```python
from build123d import *

# Parameters (mm, degrees)
F0_R     = 3
F1_DEPTH = 8
F3_DEPTH = 3
F4_R     = 2
F5_DEPTH = 25
F6_SIZE  = 0.99999
F7_R     = 4
F8_DEPTH = 1.5


# Not quite as in the source:
# - a fillet or chamfer is up to 0.001 mm smaller than in the source, because OpenCascade refuses the exact size


with BuildPart() as f1:
    # F0 (on Front) → F1 (new body)
    with BuildSketch(Plane.XZ):
        Circle(F0_R)
    extrude(amount=F1_DEPTH)

    # F2 (on face) → F3 (cut)
    with BuildSketch(Plane.XZ.offset(8)):
        Polygon((2, 1.1547005384), (0, 2.3094010768), (-2, 1.1547005384), (-2, -1.1547005384), (0, -2.3094010768), (2, -1.1547005384), align=None)
    extrude(amount=-F3_DEPTH, mode=Mode.SUBTRACT)

    # F4 (on face) → F5 (cut)
    with BuildSketch(Plane.XZ.offset(5)):
        Circle(F4_R)
    extrude(amount=-F5_DEPTH, mode=Mode.SUBTRACT)

    # F6 (size 1 in the source; OpenCascade refuses exactly that, so slightly less here)
    f6_edges = [f1.edges().sort_by_distance(p)[0] for p in [
        (-3, 0, 0),
    ]]
    chamfer(f6_edges, length=F6_SIZE)

    # F7 (on face) → F8 (join)
    with BuildSketch(Plane.XZ.offset(8)):
        Circle(F7_R)
        Polygon((2, 1.1547005384), (2, -1.1547005384), (0, -2.3094010768), (-2, -1.1547005384), (-2, 1.1547005384), (0, 2.3094010768), align=None, mode=Mode.SUBTRACT)
    extrude(amount=F8_DEPTH)


solid = f1.part
```
Could you check a few things on this model? Use its own coordinates, in mm. A direction names the side the tool comes from. Round coordinates to 2 decimals unless told otherwise and drop trailing zeros. Write each loop counter-clockwise with the first axis right and the second up, starting at its lowest first coordinate (ties: lowest second). Pieces come first, ordered by that corner, then holes.
(1) Suppose I cut it at A-A on y = -0.5. Write out the boundary of the cut face in (x, z).
Findings below:
outline: circle Ø5 at (0, 0); hole circle Ø4 at (0, 0)
(2) Thinking about a two-plate mould opening in X: for faces 1 (the face through (1, -9.5, 2)), 2 (the face through (2, -7, 0)), 3 (the face through (-0.867, -8.74, -3.905)), which applies, +X half, -X half, draft (parallel to the pull), parting line (faces both ways), or undercut?
Findings below:
face 1: draft
face 2: undercut
face 3: parting line
(3) Which directions (+Z, -Z, +X, -X, +Y, -Y) give clear straight access to the entire face, cutting with the end or side of a thin tool? Please do faces 4 (the face through (-3, -4, 0)), 5 (the face through (-2, -7, 0)), 6 (the face through (0, -3, -2)).
Findings below:
face 4: +Y
face 5: -Y
face 6: +Y, -Y
(4) If I drill on probe 1 along Z at (x, y) = (0, -3.3); probe 2 along Y at (x, z) = (2.75, -1.75); probe 3 along X at (y, z) = (-4.5, -0.5), over which ranges is the centre line in solid material (lowest first)?
Findings below:
probe 1: z = -3 to -2, 2 to 3
probe 2: y = -9.5 to -8
probe 3: x = -2.96 to -1.94, 1.94 to 2.96
(5) For pin 1 (2.5 mm diameter, centred on y = -7.5, z = 0.5, fed in from +X); pin 2 (4 mm diameter, centred on x = -3, y = -8, fed in from -Z); pin 3 (2 mm diameter, centred on x = 3, y = -5.5, fed in from +Z); pin 4 (0.5 mm diameter, centred on x = 1.5, z = -0.5, fed in from -Y), each with a flat end and sliding along its axis, tell me the tip position at first contact or that it passes through.
Findings below:
pin 1: stops at x = 4
pin 2: stops at z = -3.87
pin 3: stops at z = 2.24
pin 4: passes through
